Model file for the job. Use its own axes, mm. Face numbers are marked on the shaded views. Give positions to 0.01 mm unless a question says otherwise; leave off trailing zeros. Write each loop counter-clockwise with the first axis right and the second up, starting at its lowest first coordinate (ties: lowest second). Pieces come first, ordered by that corner, then holes.
```python
from build123d import *

# Parameters (mm, degrees)
F0_W     = 55
F0_H     = 55
F1_DEPTH = 4
F2_W     = 55
F2_H     = 55
F2_R     = 4.75
F3_DEPTH = 26
F4_R     = 5


with BuildPart() as f1:
    # F0 (on Top) → F1 (new body)
    with BuildSketch(Plane.XY):
        Rectangle(F0_W, F0_H)
    extrude(amount=F1_DEPTH)

    # F2 (on face) → F3 (join)
    with BuildSketch(Plane.XY.offset(4)):
        Rectangle(F2_W, F2_H)
        Circle(F2_R, mode=Mode.SUBTRACT)
    extrude(amount=F3_DEPTH)

    # F4
    f4_edges = [f1.edges().sort_by_distance(p)[0] for p in [
        (0, 27.5, 30),
        (-27.5, 0, 30),
        (0, -27.5, 30),
        (27.5, 0, 30),
    ]]
    fillet(f4_edges, radius=F4_R)


solid = f1.part
```
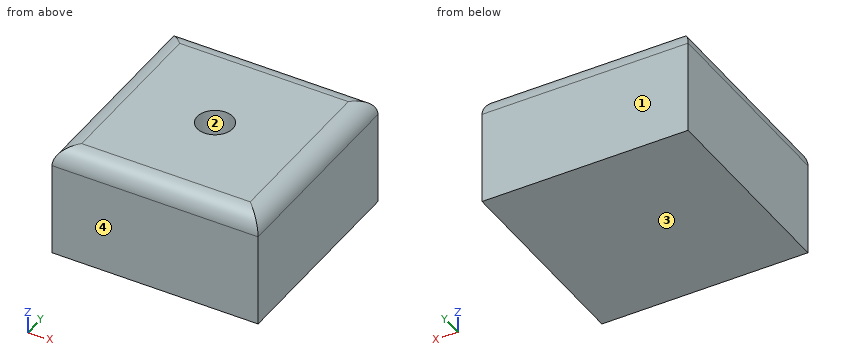
1. Pull direction Y, two halves, no side cores. Call the marked faces 1, 2, 3 and 4: +Y half, -Y half, draft (parallel to the pull), parting line (faces both ways), or undercut.
Calculated:
face 1: +Y half
face 2: undercut
face 3: draft
face 4: -Y half
2. Slice it at A-A, the plane y = 0. Write the cut outline in (x, z).
Calculated:
outline: (-27.5, 0) - (27.5, 0) - (27.5, 25) arc R5 ccw to (22.5, 30) - (4.75, 30) - (4.75, 4) - (-4.75, 4) - (-4.75, 30) - (-22.5, 30) arc R5 ccw to (-27.5, 25) - close
3. Probe probe 1 along Y at (x, z) = (0, 11.5); probe 2 along Z at (x, y) = (-2, 3.5); probe 3 along X at (y, z) = (-2, 15.25). List the from-to ranges inside material, lowest first.
Calculated:
probe 1: y = -27.5 to -4.75, 4.75 to 27.5
probe 2: z = 0 to 4
probe 3: x = -27.5 to -4.31, 4.31 to 27.5
4. Pin check, flat tips, straight feed: P1, Ø2, axis at x = 10, y = -7.5, coming from the -Z side; P2, Ø5.5, axis at x = 0, y = 0, coming from the +Z side. Stop position of each tip, or through.
Calculated:
P1: stops at z = 0
P2: stops at z = 4
5. Slice it at B-B, the plane z = 13.75. Write the cut outline in (x, y).
Calculated:
outline: (-27.5, -27.5) - (27.5, -27.5) - (27.5, 27.5) - (-27.5, 27.5) - close; hole circle Ø9.5 at (0, 0)
